```python
from build123d import *

# Parameters (mm, degrees)
SKETCH1_R           = 1.143
SKETCH1_R_2         = 0.889
BOSS_EXTRUDE1_DEPTH = 1.651
BOSS_EXTRUDE2_DEPTH = 1.8288


with BuildPart() as part:
    # Sketch1 → Boss-Extrude1 (new body)
    with BuildSketch(Plane.XY):
        with BuildLine():
            Line((-8.04553404, 11.028906935), (8.21046596, 11.028906935))
            ThreePointArc((8.21046596, 11.028906935), (9.647306939, 10.433747914), (10.24246596, 8.996906935))
            Line((10.24246596, 8.996906935), (10.24246596, -7.259093065))
            ThreePointArc((10.24246596, -7.259093065), (9.647306939, -8.695934044), (8.21046596, -9.291093065))
            Line((8.21046596, -9.291093065), (-8.04553404, -9.291093065))
            ThreePointArc((-8.04553404, -9.291093065), (-9.48237502, -8.695934044), (-10.07753404, -7.259093065))
            Line((-10.07753404, -7.259093065), (-10.07753404, 8.996906935))
            ThreePointArc((-10.07753404, 8.996906935), (-9.48237502, 10.433747914), (-8.04553404, 11.028906935))
        make_face()
        with Locations(Location((-7.53753404, 8.742906935, 0), (0, 0, 180))):
            Circle(SKETCH1_R, mode=Mode.SUBTRACT)
        with Locations(Location((7.70246596, 8.742906935, 0), (0, 0, 180))):
            Circle(SKETCH1_R, mode=Mode.SUBTRACT)
        with Locations(Location((0.08246596, -6.751093065, 0), (0, 0, 180))):
            Circle(SKETCH1_R_2, mode=Mode.SUBTRACT)
        with Locations(Location((2.62246596, -6.751093065, 0), (0, 0, 180))):
            Circle(SKETCH1_R_2, mode=Mode.SUBTRACT)
        with Locations(Location((-2.45753404, -6.751093065, 0), (0, 0, 180))):
            Circle(SKETCH1_R_2, mode=Mode.SUBTRACT)
    extrude(amount=BOSS_EXTRUDE1_DEPTH)

    # Sketch2 → Boss-Extrude2 (add)
    with BuildSketch(Plane.XY.offset(1.651)):
        with BuildLine():
            Line((2.794250427, 8.193906935), (-2.629318508, 8.193906935))
            ThreePointArc((-2.629318508, 8.193906935), (-5.41753404, 3.408906935), (-2.629318508, -1.376093065))
            Line((-2.629318508, -1.376093065), (2.794250427, -1.376093065))
            ThreePointArc((2.794250427, -1.376093065), (5.58246596, 3.408906935), (2.794250427, 8.193906935))
        make_face()
    extrude(amount=BOSS_EXTRUDE2_DEPTH)


solid = part.part
```
Can you work these out from the model? Positions are in its coordinate system, mm. A direction names the side the tool comes from. Round coordinates to 2 decimals unless told otherwise and drop trailing zeros. Loops run counter-clockwise (first coordinate to the right, second up) from the corner with the lowest first, then second, coordinate; pieces in that order, holes last.
Item 1: Suppose I cut it at D-D, the plane y = 6.5. Write out the boundary of the cut face in (x, z), then the cut area to 3 significant figures.
Item 2: Suppose I cut it at B-B, the plane x = 1.5. Write out the boundary of the cut face in (y, z).
Item 3: Will these pins go through, and if not, where does the flat tip stop? pin 1 Ø1.5 at (y, z) = (-6.5, 2.5) entering from +X; pin 2 Ø0.5 at (x, z) = (0, 3) entering from -Y; pin 3 Ø1.5 at (x, z) = (-0.5, 2.5) entering from +Y.
Item 4: Suppose I cut it at C-C, the plane z = 1.05. Write out the boundary of the cut face in (x, y), then the cut area to 3 significant figures.
Item 5: Which directions (+Z, -Z, +X, -X, +Y, -Y) give clear straight access to the entire face, cutting with the end or side of a thin tool? Please do faces 4 (the flat face through (0, -1.376, 3)), 5 (the cylindrical face through (9.663, -8.68, 0.814)), 6 (the cylindrical face through (-9.47, -8.71, 0.81)), 7 (the flat face through (0, 8.194, 3)), 8 (the cylindrical face through (-5.417, 3.49, 2.553)).
Item 6: If we mould it in two halves opening along X, with no side actions, what happens to faces 1 (the cylindrical face through (5.58, 3.33, 2.55)), 2 (the flat face through (0, 11.029, 1)), 3 (the cylindrical face through (-8.06, 9.76, 0.81))? For each: +X half, -X half, draft (parallel to the pull), parting line (faces both ways), or undercut.
Item 7: Please list where these lines run through material, in increasing order: L1, parallel to X at y = -7.5, z = 1.45; L2, parallel to Y at x = 7.5, z = 0.3; L3, parallel to Y at x = -8.5, z = 1.1.
Item 8: Suppose I cut it at A-A, the plane x = -7.75. Write out the boundary of the cut face in (y, z), then the cut area to 3 significant figures.
Reported:
1. outline: (-10.08, 0) - (10.24, 0) - (10.24, 1.65) - (4.63, 1.65) - (4.63, 3.48) - (-4.47, 3.48) - (-4.47, 1.65) - (-10.08, 1.65) - close
1. area: 50.2 mm2
2. outline: (-9.29, 0) - (11.03, 0) - (11.03, 1.65) - (8.19, 1.65) - (8.19, 3.48) - (-1.38, 3.48) - (-1.38, 1.65) - (-9.29, 1.65) - close
3. pin 1: passes through
3. pin 2: stops at y = -1.38
3. pin 3: stops at y = 8.19
4. outline: (-10.08, -7.26) arc R2.03 ccw to (-8.05, -9.29) - (8.21, -9.29) arc R2.03 ccw to (10.24, -7.26) - (10.24, 9) arc R2.03 ccw to (8.21, 11.03) - (-8.05, 11.03) arc R2.03 ccw to (-10.08, 9) - close; hole circle Ø2.29 at (-7.54, 8.74); hole circle Ø1.78 at (-2.46, -6.75); hole circle Ø1.78 at (0.08, -6.75); hole circle Ø1.78 at (2.62, -6.75); hole circle Ø2.29 at (7.7, 8.74)
4. area: 394 mm2
5. face 4: +Z, +X, -X, -Y
5. face 5: +Z, -Z, +X, -Y
5. face 6: +Z, -Z, -X, -Y
5. face 7: +Z, +X, -X, +Y
5. face 8: +Z, -X
6. face 1: +X half
6. face 2: draft
6. face 3: undercut
7. L1: x = -10.06 to -2.94, -1.98 to -0.4, 0.56 to 2.14, 3.1 to 10.23
7. L2: y = -9.29 to 7.62, 9.87 to 11.03
7. L3: y = -9.24 to 8.13, 9.36 to 10.98
8. outline: (-9.29, 0) - (7.62, 0) - (7.62, 1.65) - (-9.29, 1.65) - close; (9.87, 0) - (11.03, 0) - (11.03, 1.65) - (9.87, 1.65) - close
8. area: 29.8 mm2
